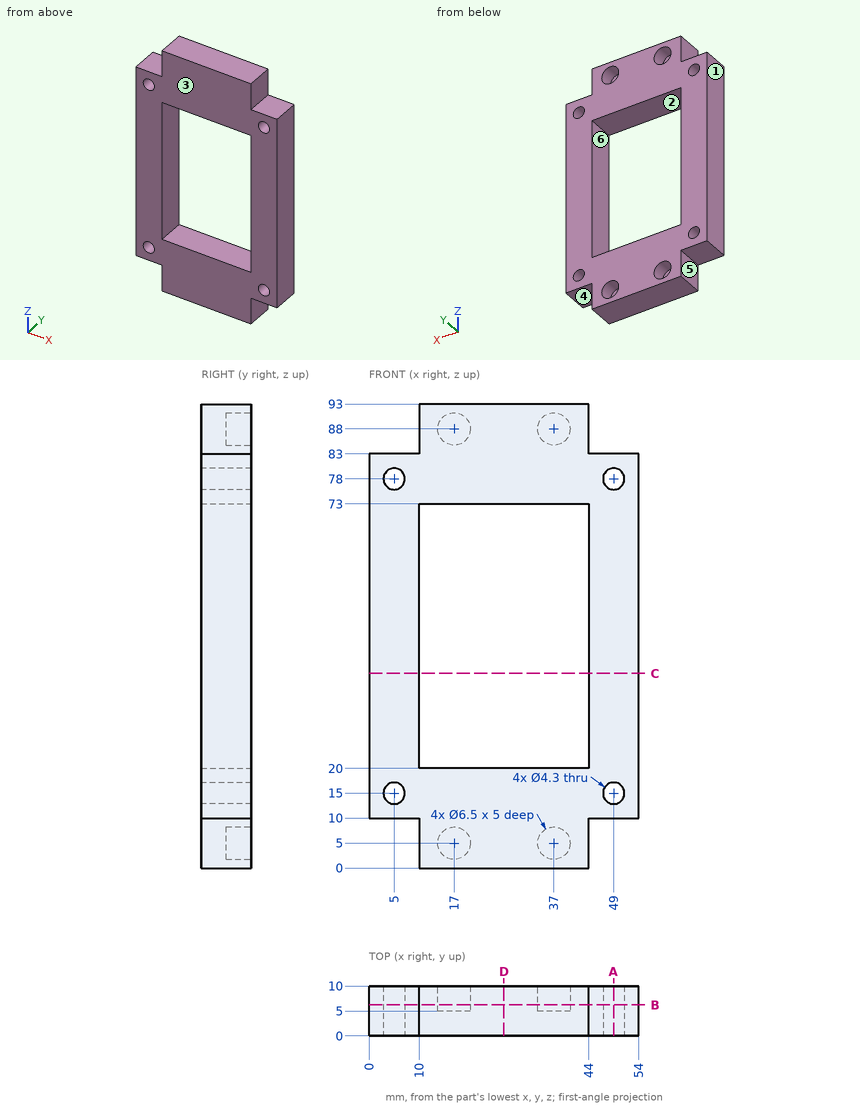
Study the drawing (mm; zero at the part's minimum x, y, z) and answer. A direction names the side the tool comes from. Give positions to 0.01 mm unless a question says otherwise; leave off trailing zeros. Write each loop counter-clockwise with the first axis right and the second up, starting at its lowest first coordinate (ties: lowest second). Pieces come first, ordered by that corner, then holes. Notation, with made-up numbers: (-16.5, -3) - (26.5, -3) arc R20 cw to (26.5, 31) - close; hole circle Ø8 at (47.25, -37.75). An arc over 180 degrees is marked (long way). One line per question, with ' | ' between items. Start each with the question number.
1. Section C-C, the plane z = 39 is taken. Determine the outline of the cut face in (x, y), then the cut area to 3 significant figures.
2. Section A-A, the plane x = 49 is taken. Determine the outline of the cut face in (y, z).
3. Straight lines are drawn through the part: line 1 (Z direction, x = 17, y = 8.65); line 2 (X direction, y = 8, z = 15); line 3 (X direction, y = 6.5, z = 43). For each, find the intervals that lie inside material, in ascending order.
4. Section B-B, the plane y = 6.25 is taken. Count the separate pieces of the cut face and the enclosed holes in it, then the cut area to 3 significant figures.
5. Section D-D, the plane x = 27 is taken. Determine the outline of the cut face in (y, z).
6. Given P1, Ø3.5, axis at x = 49, z = 78, coming from the -Y side; P2, Ø3, axis at x = 22, y = 4, coming from the -Z side; P3, Ø3, axis at x = 18, z = 87.5, coming from the +Y side, each flat-ended and moving along its own axis, determine where each tip first touches the part or whether it passes through.
7. For the marked faces 4, 5 and 6, determine the directions among +Z, -Z, +X, -X, +Y, -Y from which every point of the face is accessible in a straight line to the end or side of a thin tool.
8. Determine the mould class of the marked faces 1, 2 and 3 for opening direction X: +X half, -X half, draft (parallel to the pull), parting line (faces both ways), or undercut.
Result:
1) outline: (0, 0) - (10, 0) - (10, 10) - (0, 10) - close; (44, 0) - (54, 0) - (54, 10) - (44, 10) - close | area: 200 mm2
2) outline: (0, 10) - (10, 10) - (10, 12.85) - (0, 12.85) - close; (0, 17.15) - (10, 17.15) - (10, 75.85) - (0, 75.85) - close; (0, 80.15) - (10, 80.15) - (10, 83) - (0, 83) - close
3) line 1: z = 0 to 1.75, 8.25 to 20, 73 to 84.75, 91.25 to 93 | line 2: x = 0 to 2.85, 7.15 to 46.85, 51.15 to 54 | line 3: x = 0 to 10, 44 to 54
4) separate pieces: 1 | enclosed holes: 9 | area: 2,630 mm2
5) outline: (0, 0) - (10, 0) - (10, 20) - (0, 20) - close; (0, 73) - (10, 73) - (10, 93) - (0, 93) - close
6) P1: passes through | P2: stops at z = 0 | P3: stops at y = 5
7) face 4: -Z, +X, +Y, -Y | face 5: -Z, -X, +Y, -Y | face 6: +Y, -Y
8) face 1: -X half | face 2: undercut | face 3: draft
